```python
from build123d import *

# Parameters (mm, degrees)
SKETCH1_R           = 50
SKETCH1_R_2         = 1.5
BOSS_EXTRUDE1_DEPTH = 3
CUT_EXTRUDE1_DEPTH  = 71.774289117


with BuildPart() as part:
    # Sketch1 → Boss-Extrude1 (new body)
    with BuildSketch(Plane(origin=(0, 0, 0), x_dir=(1, 0, 0), z_dir=(0, 1, 0))):
        with Locations(Location((0, 0, 0), (0, 0, 270))):
            Circle(SKETCH1_R)
        with Locations(Location((-40, 22.5, 0), (0, 0, 270))):
            Circle(SKETCH1_R_2, mode=Mode.SUBTRACT)
        with Locations(Location((40, 22.5, 0), (0, 0, 270))):
            Circle(SKETCH1_R_2, mode=Mode.SUBTRACT)
        with Locations(Location((40, -22.5, 0), (0, 0, 270))):
            Circle(SKETCH1_R_2, mode=Mode.SUBTRACT)
        with Locations(Location((-40, -22.5, 0), (0, 0, 270))):
            Circle(SKETCH1_R_2, mode=Mode.SUBTRACT)
    extrude(amount=BOSS_EXTRUDE1_DEPTH)

    # Sketch2 → Cut-Extrude1 (cut, through all)
    with BuildSketch(Plane.XZ):
        with BuildLine():
            ThreePointArc((38.724655842, 28.361964493), (0, 48), (-38.724655842, 28.361964493))
            ThreePointArc((-38.724655842, 28.361964493), (-39.07406284, 26.796955174), (-38.161627237, 25.478319255))
            ThreePointArc((-38.161627237, 25.478319255), (-36.94948562, 20.784085661), (-41.590625258, 19.382322774))
            ThreePointArc((-41.590625258, 19.382322774), (-43.19134744, 19.477338108), (-44.347360672, 18.366044796))
            ThreePointArc((-44.347360672, 18.366044796), (-48, 0), (-44.347360672, -18.366044796))
            ThreePointArc((-44.347360672, -18.366044796), (-43.19134744, -19.477338108), (-41.590625258, -19.382322774))
            ThreePointArc((-41.590625258, -19.382322774), (-36.94948562, -20.784085661), (-38.161627237, -25.478319255))
            ThreePointArc((-38.161627237, -25.478319255), (-39.07406284, -26.796955174), (-38.724655842, -28.361964493))
            ThreePointArc((-38.724655842, -28.361964493), (0, -48), (38.724655842, -28.361964493))
            ThreePointArc((38.724655842, -28.361964493), (39.07406284, -26.796955174), (38.161627237, -25.478319255))
            ThreePointArc((38.161627237, -25.478319255), (36.94948562, -20.784085661), (41.590625258, -19.382322774))
            ThreePointArc((41.590625258, -19.382322774), (43.19134744, -19.477338108), (44.347360672, -18.366044796))
            ThreePointArc((44.347360672, -18.366044796), (48, 0), (44.347360672, 18.366044796))
            ThreePointArc((44.347360672, 18.366044796), (43.19134744, 19.477338108), (41.590625258, 19.382322774))
            ThreePointArc((41.590625258, 19.382322774), (36.94948562, 20.784085661), (38.161627237, 25.478319255))
            ThreePointArc((38.161627237, 25.478319255), (39.07406284, 26.796955174), (38.724655842, 28.361964493))
        make_face()
    extrude(amount=-CUT_EXTRUDE1_DEPTH, mode=Mode.SUBTRACT)


solid = part.part
```
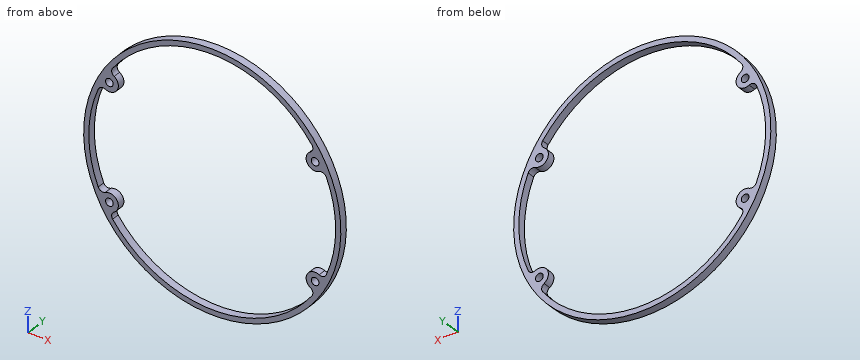
Geometry check sheet. Reference: the model listing, model coordinates, mm. Give positions to 0.01 mm unless a question says otherwise; leave off trailing zeros. Order: outer loops, then holes, each group sorted by start corner. A loop starts at its lowest first (then second) coordinate and runs counter-clockwise, first axis right, second up. Notation, with made-up numbers: (-33, 43.5) - (-16, 43.5) arc R34 cw to (-16, 77.5) - close; hole circle Ø3 at (-12.5, -15.5). An arc over 180 degrees is marked (long way). Write item = value, one per line. Start each with the question number.
1) Section check B-B (x = 0). Enter the section's corners in (y, z), then the cut area to 3 significant figures.
2) Scan lines: L1, parallel to X at y = 1.9, z = 22.5; L2, parallel to X at y = 0.3, z = -1.5; L3, parallel to X at y = 1.3, z = -44. Record each from-to range of solid material in increasing order.
3) Section check D-D (y = 1.9). Enter the section's corners in (x, z), then the cut area to 3 significant figures.
4) Section check A-A (z = 0). Enter the section's corners in (x, y).
5) Gauge pin test, flat ends, axial feed: pin 1 Ø1.5 at (x, z) = (38, -20) entering from -Y; pin 2 Ø1.5 at (x, y) = (35.5, 2.5) entering from -Z; pin 3 Ø1 at (x, y) = (-36.5, 0.5) entering from +Z. Record the tip position at first contact, or that the pin passes through.
6) Section check C-C (z = 22.5). Enter the section's corners in (x, y).
Geometry check:
q1.outline = (0, -50) - (3, -50) - (3, -48) - (0, -48) - close; (0, 48) - (3, 48) - (3, 50) - (0, 50) - close
q1.area = 12.0 mm2
q2.L1 = -44.65 to -41.5, -38.5 to -36.5, 36.5 to 38.5, 41.5 to 44.65
q2.L2 = -49.98 to -47.98, 47.98 to 49.98
q2.L3 = -23.75 to -19.18, 19.18 to 23.75
q3.outline = circle Ø100 at (0, 0); hole (-44.35, -18.37) arc R2 ccw to (-41.59, -19.38) arc R3.5 cw to (-38.16, -25.48) arc R2 ccw to (-38.72, -28.36) arc R48 ccw to (38.72, -28.36) arc R2 ccw to (38.16, -25.48) arc R3.5 cw to (41.59, -19.38) arc R2 ccw to (44.35, -18.37) arc R48 ccw to (44.35, 18.37) arc R2 ccw to (41.59, 19.38) arc R3.5 cw to (38.16, 25.48) arc R2 ccw to (38.72, 28.36) arc R48 ccw to (-38.72, 28.36) arc R2 ccw to (-38.16, 25.48) arc R3.5 cw to (-41.59, 19.38) arc R2 ccw to (-44.35, 18.37) arc R48 ccw to start; hole circle Ø3 at (-40, -22.5); hole circle Ø3 at (-40, 22.5); hole circle Ø3 at (40, -22.5); hole circle Ø3 at (40, 22.5)
q3.area = 731 mm2
q4.outline = (-50, 0) - (-48, 0) - (-48, 3) - (-50, 3) - close; (48, 0) - (50, 0) - (50, 3) - (48, 3) - close
q5.pin_1 = 0
q5.pin_2 = -35.95
q5.pin_3 = 34.7
q6.outline = (-44.65, 0) - (-41.5, 0) - (-41.5, 3) - (-44.65, 3) - close; (-38.5, 0) - (-36.5, 0) - (-36.5, 3) - (-38.5, 3) - close; (36.5, 0) - (38.5, 0) - (38.5, 3) - (36.5, 3) - close; (41.5, 0) - (44.65, 0) - (44.65, 3) - (41.5, 3) - close
